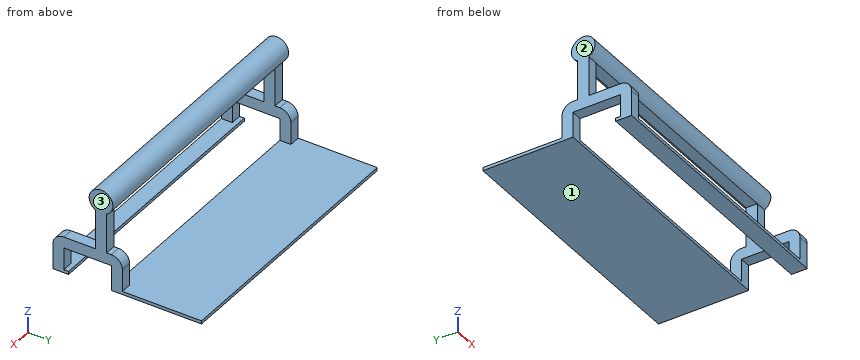
```python
from build123d import *

# Parameters (mm, degrees)
PAD_DEPTH    = 170
SKETCH001_W  = 46
SKETCH001_H  = 156
POCKET_DEPTH = 44.001


with BuildPart() as part:
    # Sketch → Pad (new body)
    with BuildSketch(Plane.YZ):
        with BuildLine():
            Line((7, 0), (27, 0))
            Line((27, 0), (27, 25))
            ThreePointArc((34, 25), (30.5, 39.13325), (27, 25))
            Line((34, 25), (34, 0))
            Line((34, 0), (37, 0))
            ThreePointArc((44, -7), (41.949747, -2.050253), (37, 0))
            Line((44, -7), (44, -21))
            Line((44, -21), (94, -21))
            Line((94, -21), (94, -23))
            Line((94, -23), (37, -23))
            Line((37, -23), (37, -7))
            Line((37, -7), (7, -7))
            Line((7, -7), (7, -21))
            Line((7, -21), (10, -21))
            Line((10, -21), (10, -23))
            Line((10, -23), (0, -23))
            Line((0, -23), (0, -7))
            ThreePointArc((7, 0), (2.050253, -2.050253), (0, -7))
        make_face()
    extrude(amount=PAD_DEPTH)

    # Sketch001 (on Face7 of Pad) → Pocket (cut, through all)
    with BuildSketch(Plane.ZX.offset(44)):
        with Locations((2, 85)):
            Rectangle(SKETCH001_W, SKETCH001_H)
    extrude(amount=-POCKET_DEPTH, mode=Mode.SUBTRACT)


solid = part.part
```
Build history of the part. All positions in model axes, mm. Face numbers are marked on the shaded views. Round coordinates to 2 decimals unless told otherwise and drop trailing zeros. Order: outer loops, then holes, each group sorted by start corner. A loop starts at its lowest first (then second) coordinate and runs counter-clockwise, first axis right, second up. Notation, with made-up numbers: (53, 34) -> (103, 34) arc R21 cw to (103, 59) -> close; hole circle Ø10 at (71, 57). An arc over 180 degrees is marked (long way). Answer in a Markdown table with one row per item.
1) Wall check: L1, parallel to Z at x = 48.5, y = 84; L2, parallel to Y at x = 150, z = 31; L3, parallel to Z at x = 143.5, y = 24.5. Give the ranges that are in metal, low to high.
Values:
| item | result |
|---|---|
| L1 | -23 to -21 |
| L2 | 23.03 to 37.97 |
| L3 | 27.13 to 36.13 |
2) Pin check, flat tips, straight feed: P1, Ø3.5, axis at x = 167, y = 35, coming from the +Z side; P2, Ø3.5, axis at x = 2, y = 35.5, coming from the +Z side; P3, Ø5.5, axis at x = 72.5, y = 29, coming from the -Z side. Stop position of each tip, or through.
Values:
| item | result |
|---|---|
| P1 | z = 38.61 |
| P2 | z = 38.39 |
| P3 | z = 25 |
3) Mould opens along X. For the marked faces 1, 2 and 3 say: released by +X, released by -X, zero draft, split by the parting line, or undercut.
Values:
| item | result |
|---|---|
| face 1 | zero draft |
| face 2 | released by -X |
| face 3 | released by +X |
4) Band-saw the part on A-A on x = 17.5. Give the cut face in (y, z).
Values:
| item | result |
|---|---|
| outline | (0, -23) -> (10, -23) -> (10, -21) -> (0, -21) -> close; (27, 25) -> (34, 25) arc R7.5 ccw (long way) to start; (37, -23) -> (94, -23) -> (94, -21) -> (37, -21) -> close |
5) Band-saw the part on B-B on y = 30.5. Give the cut face in (x, z).
Values:
| item | result |
|---|---|
| outline | (0, -7) -> (7, -7) -> (7, 25) -> (163, 25) -> (163, -7) -> (170, -7) -> (170, 39.13) -> (0, 39.13) -> close |
6) Band-saw the part on D-D on y = 78.5. Give the cut face in (x, z).
Values:
| item | result |
|---|---|
| outline | (0, -23) -> (170, -23) -> (170, -21) -> (0, -21) -> close |
7) Band-saw the part on C-C on z = -4.5. Give the cut face in (x, y).
Values:
| item | result |
|---|---|
| outline | (0, 0.46) -> (7, 0.46) -> (7, 43.54) -> (0, 43.54) -> close; (163, 0.46) -> (170, 0.46) -> (170, 43.54) -> (163, 43.54) -> close |
